from build123d import *

# Parameters (mm, degrees)
SKETCH1_R           = 10
SKETCH1_R_2         = 5.1
BOSS_EXTRUDE1_DEPTH = 4
SKETCH3_R           = 3
BOSS_EXTRUDE2_DEPTH = 12
SKETCH4_R           = 10
SKETCH4_R_2         = 3
BOSS_EXTRUDE3_DEPTH = 2
CHAMFER2_SIZE       = 1
CHAMFER4_SIZE       = 0.5
CUT_EXTRUDE1_REACH  = 8
SKETCH5_R           = 0.75


with BuildPart() as part:
    # Sketch1 → Boss-Extrude1 (new body)
    with BuildSketch(Plane.XY):
        Circle(SKETCH1_R)
        Circle(SKETCH1_R_2, mode=Mode.SUBTRACT)
    extrude(amount=BOSS_EXTRUDE1_DEPTH)



with BuildPart() as body_2:
    # Sketch3 → Boss-Extrude2 (new body)
    with BuildSketch(Plane(origin=(0, 0, 0), x_dir=(-1, 0, 0), z_dir=(0, 0, -1))):
        Circle(SKETCH3_R)
    extrude(amount=BOSS_EXTRUDE2_DEPTH)


with BuildPart() as part_1:
    add(part.part)

    add(body_2.part)  # Boss-Extrude3 merges body 2
    # Sketch4 → Boss-Extrude3 (add)
    with BuildSketch(Plane(origin=(0, 0, 0), x_dir=(-1, 0, 0), z_dir=(0, 0, -1))):
        Circle(SKETCH4_R)
        Circle(SKETCH4_R_2, mode=Mode.SUBTRACT)
    extrude(amount=BOSS_EXTRUDE3_DEPTH)

    # Chamfer2
    chamfer2_edges = [part_1.edges().sort_by_distance(p)[0] for p in [
        (3, 0, -2),
    ]]
    chamfer(chamfer2_edges, length=CHAMFER2_SIZE)

    # Chamfer4
    chamfer4_edges = [part_1.edges().sort_by_distance(p)[0] for p in [
        (3, 0, -12),
    ]]
    chamfer(chamfer4_edges, length=CHAMFER4_SIZE)

    # Sketch5 → Cut-Extrude1 (cut, up to next)
    with BuildSketch(Plane(origin=(0, 0, -2), x_dir=(-1, 0, 0), z_dir=(0, 0, -1)), mode=Mode.PRIVATE) as cut_extrude1_sk1:
        with Locations((-8.5, 0)):
            Circle(SKETCH5_R)
    cut_extrude1_tool1 = extrude(cut_extrude1_sk1.sketch, amount=-CUT_EXTRUDE1_REACH, mode=Mode.PRIVATE) & part_1.part
    add(cut_extrude1_tool1.solids().sort_by_distance((8.5, 0, -2))[0], mode=Mode.SUBTRACT)
    # Sketch5 → Cut-Extrude1 (cut, up to next)
    with BuildSketch(Plane(origin=(0, 0, -2), x_dir=(-1, 0, 0), z_dir=(0, 0, -1)), mode=Mode.PRIVATE) as cut_extrude1_sk2:
        with Locations((6.5, 0)):
            Circle(SKETCH5_R)
    cut_extrude1_tool2 = extrude(cut_extrude1_sk2.sketch, amount=-CUT_EXTRUDE1_REACH, mode=Mode.PRIVATE) & part_1.part
    add(cut_extrude1_tool2.solids().sort_by_distance((-6.5, 0, -2))[0], mode=Mode.SUBTRACT)


solid = part_1.part
Geometry check sheet. Reference: the model listing, model coordinates, mm. A direction names the side the tool comes from. Give positions to 0.01 mm unless a question says otherwise; leave off trailing zeros. Write each loop counter-clockwise with the first axis right and the second up, starting at its lowest first coordinate (ties: lowest second). Pieces come first, ordered by that corner, then holes. Notation, with made-up numbers: (26.5, -24) - (81.5, -24) arc R4 ccw to (81.5, -19) - close; hole circle Ø10 at (-0.5, 76). An arc over 180 degrees is marked (long way). Put each result on its own line as item: value.
1. Sectioned sample at B-B, the plane x = 0. Enter the section's corners in (y, z), plus the area to 3 significant figures.
Ans:
outline: (-10, -2) - (-4, -2) - (-3, -3) - (-3, -11.5) - (-2.5, -12) - (2.5, -12) - (3, -11.5) - (3, -3) - (4, -2) - (10, -2) - (10, 4) - (5.1, 4) - (5.1, 0) - (-5.1, 0) - (-5.1, 4) - (-10, 4) - close
area: 140 mm²
2. Thickness scan on line 1 (Y direction, x = 0, z = 2.1); line 2 (Z direction, x = -4.5, y = -4.75); line 3 (Z direction, x = 2, y = -0.5). Record the ranges inside material, lowest first.
Ans:
line 1: y = -10 to -5.1, 5.1 to 10
line 2: z = -2 to 4
line 3: z = -12 to 0
3. Sectioned sample at A-A, the plane y = 0. Enter the section's corners in (x, z).
Ans:
outline: (-10, -2) - (-7.25, -2) - (-7.25, 4) - (-10, 4) - close; (-5.75, -2) - (-4, -2) - (-3, -3) - (-3, -11.5) - (-2.5, -12) - (2.5, -12) - (3, -11.5) - (3, -3) - (4, -2) - (7.75, -2) - (7.75, 4) - (5.1, 4) - (5.1, 0) - (-5.1, 0) - (-5.1, 4) - (-5.75, 4) - close; (9.25, -2) - (10, -2) - (10, 4) - (9.25, 4) - close
4. Set-up check for faces 4 (the flat face through (-5, 2, 4)), 5 (the cylindrical face through (2.4, -4.5, 2)): record each of +Z, -Z, +X, -X, +Y, -Y from which the full face is reachable in a straight line by a thin tool's end or side.
Ans:
face 4: +Z, +X, -X, +Y, -Y
face 5: +Z
5. Go/stop test with flat-tipped pins: pin 1 (1 mm diameter, centred on x = 4.5, z = -8, fed in from -Y); pin 2 (3 mm diameter, centred on x = 5.5, y = 4, fed in from -Z); pin 3 (2 mm diameter, centred on y = 6.5, z = 1.5, fed in from +X); pin 4 (1.8 mm diameter, centred on x = 1.5, y = -1, fed in from +Z). Record where each tip stops, or that it passes through.
Ans:
pin 1: passes through
pin 2: stops at z = -2
pin 3: stops at x = 8.35
pin 4: stops at z = 0
6. Draft check along X on faces 1 (the cylindrical face through (3, 0, -7)), 2 (the cylindrical face through (9.25, 0.03, 0.96)), 3 (the flat face through (-4.3, 0.1, -2)). Enter one of: +X half, -X half, draft (parallel to the pull), parting line (faces both ways), or undercut.
Ans:
face 1: parting line
face 2: undercut
face 3: draft
7. Sectioned sample at D-D, the plane z = -1. Enter the section's corners in (x, y).
Ans:
outline: circle Ø20 at (0, 0); hole circle Ø1.5 at (-6.5, 0); hole circle Ø1.5 at (8.5, 0)
8. Sectioned sample at C-C, the plane x = 8.75. Enter the section's corners in (y, z), plus the area to 3 significant figures.
Ans:
outline: (-4.84, -2) - (-0.71, -2) - (-0.71, 4) - (-4.84, 4) - close; (0.71, -2) - (4.84, -2) - (4.84, 4) - (0.71, 4) - close
area: 49.6 mm²
